The listing builds one solid part. Answer for the finished solid, in the listing's coordinates (mm). A direction names the side the tool comes from. Coordinates: 2 decimals unless noted, no trailing zeros. Loops run counter-clockwise (first coordinate to the right, second up) from the corner with the lowest first, then second, coordinate; pieces in that order, holes last. Notation, with made-up numbers: M -26,-25.75 L 0,-25.75 A21 ccw 0,-21.75 Z; hole C -23,49 d11. An arc over 180 degrees is marked long. Return JSON: item names as keys, results as strings. Group by question number.
1. Section A-A (x = 234) is taken. Write down the section's boundary in (y, z).
2. Section C-C (z = 261) is taken. Write down the section's boundary in (x, y), then the cut area to 3 significant figures.
3. Section D-D (x = 515.5) is taken. Write down the section's boundary in (y, z), then the cut area to 3 significant figures.
4. The mould has two halves that part along Z. Classify faces 6 (the face through (296, -350.839, 19)), 7 (the face through (296, -154, -42.149)), 8 (the face through (297.2, 164.566, 333.707)): pulls with the +Z half, pulls with the -Z half, needs draft (parallel to the pull), parting line crosses it, or undercut.
5. Section B-B (y = 155) is taken. Write down the section's boundary in (x, z), then the cut area to 3 significant figures.
6. Given P1, Ø8, axis at x = 280.5, y = -253.5, coming from the +Z side; P2, Ø5, axis at x = 159.5, y = -184.5, coming from the +Z side; P3, Ø10, axis at x = 184, y = -194.5, coming from the +Z side, each flat-ended and moving along its own axis, determine where each tip first touches the part or whether it passes through.
7. Straight lines are drawn through the part: L1, parallel to Y at x = 415.5, z = -449.5; L2, parallel to Z at x = 274.5, y = 42; L3, parallel to Z at x = 249, y = 2. For each, find the intervals that lie inside material, in ascending order. Write a range as from..to.
8. Which of the six approach directions +Z, -Z, +X, -X, +Y, -Y give full straight-line access (tool end or side, diameter ignored) to faces 1 (the face through (296, 296, -542.149)), 2 (the face through (500, 165, 329)), 3 (the face through (296, 49.161, -289)), 4 (the face through (100, 165, 329)), 5 (the face through (296, 275.498, 598))?
```python
from build123d import *

# Parameters (mm, degrees)
F1_DEPTH = 600
F2_W     = 400
F2_H     = 260
F3_DEPTH = 5
F4_SIZE  = 20


with BuildPart() as f1:
    # F0 (on Right) → F1 (new body)
    with BuildSketch(Plane.YZ):
        Polygon((549.161103, 657.850861), (275.498464, 657.850861), (275.498464, 557.850861), (49.158994, 76.551717), (-350.838897, 77.850861), (-350.838897, -42.149139), (49.161103, -42.149139), (49.161103, -542.149139), (549.161103, -542.149139), align=None)
    extrude(amount=F1_DEPTH)

    # F2 (on face) → F3 (join)
    with BuildSketch(Plane(origin=(0, 10.776047, -5.067628), x_dir=(1, 0, 0), z_dir=(0, -0.90493, 0.42556))):
        with Locations((300, 370.194057)):
            Rectangle(F2_W, F2_H)
    extrude(amount=F3_DEPTH)

    # F4
    f4_edges = [f1.edges().sort_by_distance(p)[0] for p in [
        (300, 275.498464, 657.850861),
        (300, 549.161103, 657.850861),
        (600, -350.838897, 17.850861),
        (0, -350.838897, 17.850861),
    ]]
    chamfer(f4_edges, length=F4_SIZE)


solid = f1.part
```
Worked out:
{
 "1": {"outline": "M -350.84,-42.15 L 49.16,-42.15 L 49.16,-542.15 L 549.16,-542.15 L 549.16,637.85 L 529.16,657.85 L 295.5,657.85 L 275.5,637.85 L 275.5,557.85 L 223.64,447.57 L 219.11,449.7 L 108.47,214.42 L 112.99,212.29 L 49.16,76.55 L -350.84,77.85 Z"},
 "2": {"outline": "M 0,135.9 L 100,135.9 L 100,130.37 L 500,130.37 L 500,135.9 L 600,135.9 L 600,549.16 L 0,549.16 Z", "area": "250,000 mm^2"},
 "3": {"outline": "M -350.84,-42.15 L 49.16,-42.15 L 49.16,-542.15 L 549.16,-542.15 L 549.16,637.85 L 529.16,657.85 L 295.5,657.85 L 275.5,637.85 L 275.5,557.85 L 49.16,76.55 L -350.84,77.85 Z", "area": "570,000 mm^2"},
 "4": {"face 6": "needs draft", "face 7": "pulls with the -Z half", "face 8": "pulls with the +Z half"},
 "5": {"outline": "M 0,-542.15 L 600,-542.15 L 600,301.62 L 500,301.62 L 500,313.37 L 100,313.37 L 100,301.62 L 0,301.62 Z", "area": "511,000 mm^2"},
 "6": {"P1": "z = 77.55", "P2": "z = 77.32", "P3": "z = 77.36"},
 "7": {"L1": "49.16..549.16", "L2": "-42.15..76.57", "L3": "-42.15..76.7"},
 "8": {"face 1": "-Z, +X, -X, +Y, -Y", "face 2": "+Z, +X, -Y", "face 3": "-Z, +X, -X, -Y", "face 4": "+Z, -X, -Y", "face 5": "+Z, +X, -X, -Y"}
}
